```python
from build123d import *

# Parameters (mm, degrees)
SKIZZE1_W                       = 26.5
SKIZZE1_H                       = 61.5
AUFSATZ_LINEAR_AUSTRAGEN1_DEPTH = 1.5
SKIZZE2_R                       = 1.55
SCHNITT_LINEAR_AUSTRAGEN1_DEPTH = 2.5
SKIZZE3_W                       = 10
SKIZZE3_H                       = 8
AUFSATZ_LINEAR_AUSTRAGEN2_DEPTH = 10
SKIZZE4_R                       = 1.5
AUFSATZ_LINEAR_AUSTRAGEN3_DEPTH = 4


with BuildPart() as part:
    # Skizze1 → Aufsatz-Linear austragen1 (new body)
    with BuildSketch(Plane(origin=(0, 0, 0), x_dir=(1, 0, 0), z_dir=(0, 1, 0))):
        Rectangle(SKIZZE1_W, SKIZZE1_H)
    extrude(amount=AUFSATZ_LINEAR_AUSTRAGEN1_DEPTH)

    # Skizze2 → Schnitt-Linear austragen1 (cut, through all)
    with BuildSketch(Plane(origin=(0, 1.5, 0), x_dir=(1, 0, 0), z_dir=(0, 1, 0))):
        with Locations((-10.75, 28.25)):
            Circle(SKIZZE2_R)
        with Locations((11.25, 28.25)):
            Circle(SKIZZE2_R)
        with Locations((11.25, -28.45)):
            Circle(SKIZZE2_R)
        with Locations((-10.75, -28.45)):
            Circle(SKIZZE2_R)
    extrude(amount=-SCHNITT_LINEAR_AUSTRAGEN1_DEPTH, mode=Mode.SUBTRACT)

    # Skizze3 → Aufsatz-Linear austragen2 (add)
    with BuildSketch(Plane(origin=(0, 1.5, 0), x_dir=(1, 0, 0), z_dir=(0, 1, 0))):
        with Locations((0, -26.75)):
            Rectangle(SKIZZE3_W, SKIZZE3_H)
        with Locations((0, 26.75)):
            Rectangle(SKIZZE3_W, SKIZZE3_H)
    extrude(amount=AUFSATZ_LINEAR_AUSTRAGEN2_DEPTH)

    # Skizze4 → Aufsatz-Linear austragen3 (add)
    with BuildSketch(Plane(origin=(0, 0, -30.75), x_dir=(-1, 0, 0), z_dir=(0, 0, -1))):
        with Locations((-2, 6.5)):
            Circle(SKIZZE4_R)
        with Locations((2, 6.5)):
            Circle(SKIZZE4_R)
    extrude(amount=AUFSATZ_LINEAR_AUSTRAGEN3_DEPTH)


solid = part.part
```
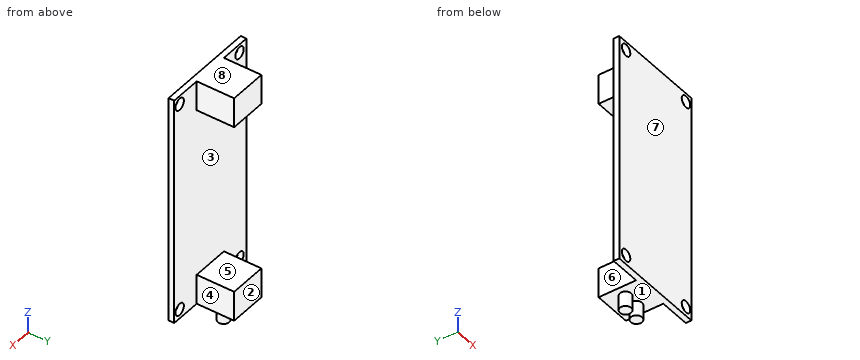
Geometry check sheet. Reference: the model listing, model coordinates, mm. Face numbers are marked on the shaded views. A direction names the side the tool comes from. Round coordinates to 2 decimals unless told otherwise and drop trailing zeros. Order: outer loops, then holes, each group sorted by start corner. A loop starts at its lowest first (then second) coordinate and runs counter-clockwise, first axis right, second up. Notation, with made-up numbers: (-16, 42.5) -> (-4, 42.5) arc R19 cw to (-4, 55.5) -> close; hole circle Ø11 at (67, 31). An arc over 180 degrees is marked (long way). Return JSON: item names as keys, results as strings. Group by question number.
Q1. Section check A-A, the plane y = 2.5. Record the boundary of the cut face in (x, z).
Q2. Material ranges on probe 1 along X at (y, z) = (1.25, -28.25); probe 2 along Z at (x, y) = (11.25, 0.65); probe 3 along Z at (x, y) = (-0.75, 6.75), recorded low to high. Write a range as from..to.
Q3. Section check D-D, the plane x = -11.5. Record the boundary of the cut face in (y, z), plus the area to 3 significant figures.
Q4. Section check C-C, the plane x = 2. Record the boundary of the cut face in (y, z).
Q5. Tool access check on the marked faces 4, 5, 6, 7 and 8. Record the directions out of +Z, -Z, +X, -X, +Y, -Y that give a thin tool (end or side, any length) a straight path to the whole face; none if there is none.
Q6. Gauge pin test, flat ends, axial feed: pin 1 (2.5 mm diameter, centred on y = 6.5, z = -28.5, fed in from +X); pin 2 (6 mm diameter, centred on x = -6, z = -9.5, fed in from +Y); pin 3 (6.5 mm diameter, centred on y = 7, z = -28, fed in from -X). Record the tip position at first contact, or that the pin passes through.
Q7. Section check B-B, the plane z = -28.25. Record the boundary of the cut face in (x, y).
Q8. Release check for a two-part mould opening along Z. For the marked faces 1, 2 and 3 record: released by +Z, released by -Z, zero draft, split by the parting line, or undercut.
Numbers:
{
 "1": {"outline": "(-5, -30.75) -> (5, -30.75) -> (5, -22.75) -> (-5, -22.75) -> close; (-5, 22.75) -> (5, 22.75) -> (5, 30.75) -> (-5, 30.75) -> close"},
 "2": {"probe 1": "-13.25..-12.3, -9.2..9.7, 12.8..13.25", "probe 2": "-30.75..-29.8, -26.7..26.9, 30..30.75", "probe 3": "-34.75..-22.75, 22.75..30.75"},
 "3": {"outline": "(0, -30.75) -> (1.5, -30.75) -> (1.5, -29.61) -> (0, -29.61) -> close; (0, -26.89) -> (1.5, -26.89) -> (1.5, 27.09) -> (0, 27.09) -> close; (0, 29.81) -> (1.5, 29.81) -> (1.5, 30.75) -> (0, 30.75) -> close", "area": "84.1 mm^2"},
 "4": {"outline": "(0, -30.75) -> (5, -30.75) -> (5, -34.75) -> (8, -34.75) -> (8, -30.75) -> (11.5, -30.75) -> (11.5, -22.75) -> (1.5, -22.75) -> (1.5, 22.75) -> (11.5, 22.75) -> (11.5, 30.75) -> (0, 30.75) -> close"},
 "5": {"face 4": "+Z, -Z, +X, +Y", "face 5": "+X, -X, +Y", "face 6": "+Z, -Z, -X, +Y", "face 7": "+Z, -Z, +X, -X, -Y", "face 8": "+Z, +X, -X, +Y, -Y"},
 "6": {"pin 1": "x = 5", "pin 2": "y = 1.5", "pin 3": "x = -5"},
 "7": {"outline": "(-13.25, 0) -> (-12.3, 0) -> (-12.3, 1.5) -> (-13.25, 1.5) -> close; (-9.2, 0) -> (9.7, 0) -> (9.7, 1.5) -> (5, 1.5) -> (5, 11.5) -> (-5, 11.5) -> (-5, 1.5) -> (-9.2, 1.5) -> close; (12.8, 0) -> (13.25, 0) -> (13.25, 1.5) -> (12.8, 1.5) -> close"},
 "8": {"face 1": "released by -Z", "face 2": "zero draft", "face 3": "undercut"}
}
